```python
from build123d import *

# Parameters (mm, degrees)
F1_DEPTH = 9.525
F2_R     = 1.98374
F3_R     = 3.69316
F4_R     = 2.15265
F5_DEPTH = 1.70942
F6_R     = 2.15265
F7_DEPTH = 1.70942
F8_R     = 0.79375


with BuildPart() as f1:
    # F0 (on Top) → F1 (new body)
    with BuildSketch(Plane.XY):
        Polygon((0, 20.51558), (0, 0), (-20.51558, 0), (-20.51558, -1.70942), (1.70942, -1.70942), (1.70942, 20.51558), align=None)
    extrude(amount=F1_DEPTH)

    # F2
    f2_edges = [f1.edges().sort_by_distance(p)[0] for p in [
        (0, 0, 4.7625),
    ]]
    fillet(f2_edges, radius=F2_R)

    # F3
    f3_edges = [f1.edges().sort_by_distance(p)[0] for p in [
        (1.70942, -1.70942, 4.7625),
    ]]
    fillet(f3_edges, radius=F3_R)

    # F4 (on face) → F5 (cut, through all)
    with BuildSketch(Plane(origin=(0, 0, 0), x_dir=(-1, 0, 0), z_dir=(0, 1, 0))):
        with Locations((15.75308, 4.7625)):
            Circle(F4_R)
    extrude(amount=-F5_DEPTH, mode=Mode.SUBTRACT)

    # F6 (on face) → F7 (cut, through all)
    with BuildSketch(Plane(origin=(0, 0, 0), x_dir=(0, -1, 0), z_dir=(-1, 0, 0))):
        with Locations((-15.75308, 4.7625)):
            Circle(F6_R)
    extrude(amount=-F7_DEPTH, mode=Mode.SUBTRACT)

    # F8
    f8_edges = [f1.edges().sort_by_distance(p)[0] for p in [
        (0.85471, 20.51558, 0),
        (0.85471, 20.51558, 9.525),
        (-20.51558, -0.85471, 9.525),
        (-20.51558, -0.85471, 0),
    ]]
    fillet(f8_edges, radius=F8_R)


solid = f1.part
```
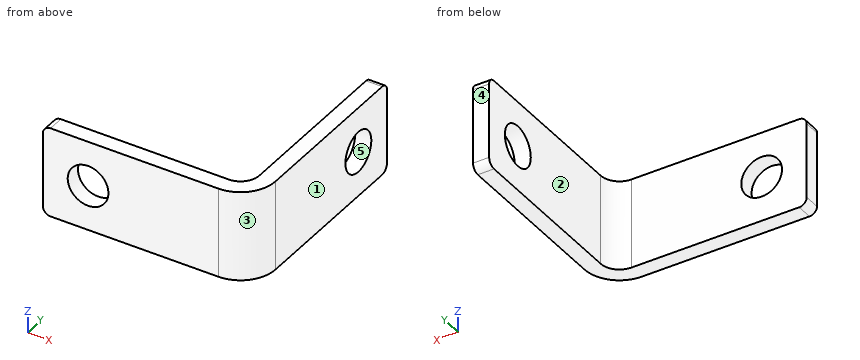
Source: CAD feature listing. Evaluate the final solid. Frame: model axes, mm. Face numbers are marked on the shaded views. A direction names the side the tool comes from. Round coordinates to 2 decimals unless told otherwise and drop trailing zeros. Loops run counter-clockwise (first coordinate to the right, second up) from the corner with the lowest first, then second, coordinate; pieces in that order, holes last.
(1) Section query B-B (z = 2). Output: boundary loops of the cut face in (x, y), and give its area (3 significant figures).
From the geometry:
outline: (-20.52, -1.71) - (-1.98, -1.71) arc R3.69 ccw to (1.71, 1.98) - (1.71, 20.52) - (0, 20.52) - (0, 1.98) arc R1.98 cw to (-1.98, 0) - (-20.52, 0) - close
area: 71.0 mm2
(2) Access query for the marked faces 1 and 2. Directions: +Z, -Z, +X, -X, +Y, -Y. A direction counts if a zero-diameter tool reaches every point of the face in a straight line with its end or side. Return the directions, or none.
From the geometry:
face 1: +Z, -Z, +X, +Y, -Y
face 2: +Z, -Z, -X, +Y
(3) Section query A-A (z = 5.5). Output: boundary loops of the cut face in (x, y), and give its area (3 significant figures).
From the geometry:
outline: (-20.52, -1.71) - (-17.78, -1.71) - (-17.78, 0) - (-20.52, 0) - close; (-13.73, -1.71) - (-1.98, -1.71) arc R3.69 ccw to (1.71, 1.98) - (1.71, 13.73) - (0, 13.73) - (0, 1.98) arc R1.98 cw to (-1.98, 0) - (-13.73, 0) - close; (0, 17.78) - (1.71, 17.78) - (1.71, 20.52) - (0, 20.52) - close
area: 57.2 mm2
(4) Section query D-D (y = 14.5). Output: boundary loops of the cut face in (x, z) (3 decimals).
From the geometry:
outline: (0, 0) - (1.709, 0) - (1.709, 3.012) - (0, 3.012) - close; (0, 6.513) - (1.709, 6.513) - (1.709, 9.525) - (0, 9.525) - close
(5) Section query C-C (x = -14.5). Output: boundary loops of the cut face in (y, z) (3 decimals).
From the geometry:
outline: (-1.709, 0) - (0, 0) - (0, 3.012) - (-1.709, 3.012) - close; (-1.709, 6.513) - (0, 6.513) - (0, 9.525) - (-1.709, 9.525) - close
(6) Pull-direction query (Y, two-part tool) for the marked faces 3, 4 and 5; classes: +Y half, -Y half, draft (parallel to the pull), parting line (faces both ways), or undercut.
From the geometry:
face 3: -Y half
face 4: +Y half
face 5: undercut
(7) Contact query for flat-ended pins moving along their axis: pin 1 Ø12 at (x, y) = (-14.5, 7.5) entering from -Z; pin 2 Ø5 at (y, z) = (7, 3) entering from -X. Output: stop coordinate, or through.
From the geometry:
pin 1: passes through
pin 2: stops at x = 0
(8) Material intervals for probe 1 along Y at (x, z) = (-14.75, 2.75); probe 2 along X at (y, z) = (6.25, 2); probe 3 along Y at (x, z) = (0.75, 5.75), sorted ascending.
From the geometry:
probe 1: y = -1.71 to 0
probe 2: x = 0 to 1.71
probe 3: y = -0.5 to 13.84, 17.67 to 20.52
